```python
from build123d import *

# Parameters (mm, degrees)
SKETCH1_R          = 12.5
SKETCH1_R_2        = 1.5
SKETCH1_R_3        = 2.5
SKETCH1_R_4        = 2.25
BASE_FLANGE1_DEPTH = 1


# Sheet-metal steps are written as plain solids
with BuildPart() as part:
    # Sketch1 → Base-Flange1 (new body)
    with BuildSketch(Plane.XY):
        Polygon((-90.1, -21), (-48.1, -21), (-30.1, -50), (-20.1, -50), (4.727586207, -10), (90.1, -10), (90.1, 10), (4.727586207, 10), (-20.1, 50), (-30.1, 50), (-48.1, 21), (-90.1, 21), align=None)
        with Locations((-69.1, 0)):
            Circle(SKETCH1_R, mode=Mode.SUBTRACT)
        with Locations((-84.6, 15.5)):
            Circle(SKETCH1_R_2, mode=Mode.SUBTRACT)
        with Locations((-25.1, -40)):
            Circle(SKETCH1_R_3, mode=Mode.SUBTRACT)
        with Locations((80.1, 0)):
            Circle(SKETCH1_R_4, mode=Mode.SUBTRACT)
        with Locations((65.1, 0)):
            Circle(SKETCH1_R_4, mode=Mode.SUBTRACT)
        with Locations((25.1, 0)):
            Circle(SKETCH1_R_4, mode=Mode.SUBTRACT)
        with Locations((5.1, 0)):
            Circle(SKETCH1_R_4, mode=Mode.SUBTRACT)
        with Locations((36.1, 0)):
            Circle(SKETCH1_R_3, mode=Mode.SUBTRACT)
        with Locations(Location((-25.1, 40, 0), (0, 0, 180))):
            Circle(SKETCH1_R_3, mode=Mode.SUBTRACT)
        with Locations((-15.1, 0)):
            Circle(SKETCH1_R_4, mode=Mode.SUBTRACT)
        with Locations((-35.1, 0)):
            Circle(SKETCH1_R_4, mode=Mode.SUBTRACT)
        with Locations((-53.6, 15.5)):
            Circle(SKETCH1_R_2, mode=Mode.SUBTRACT)
        with Locations((-53.6, -15.5)):
            Circle(SKETCH1_R_2, mode=Mode.SUBTRACT)
        with Locations((-84.6, -15.5)):
            Circle(SKETCH1_R_2, mode=Mode.SUBTRACT)
    extrude(amount=-BASE_FLANGE1_DEPTH)


solid = part.part
```
Source: CAD feature listing. Evaluate the final solid. Frame: model axes, mm. Give positions to 0.01 mm unless a question says otherwise; leave off trailing zeros. Loops run counter-clockwise (first coordinate to the right, second up) from the corner with the lowest first, then second, coordinate; pieces in that order, holes last. Notation, with made-up numbers: (20.25, -10.75) - (78.25, -10.75) arc R25 ccw to (78.25, 2.25) - close; hole circle Ø1 at (9, 72.25). An arc over 180 degrees is marked (long way). Use CSV: the item, a comma, the result in double quotes. Start each with the question number.
1. Ray query, L1, parallel to Y at x = -25.1, z = -0.25; L2, parallel to Y at x = 57, z = -0.6; L3, parallel to Y at x = -35.1, z = -0.75. Return the intervals inside material, ascending.
2. Section C-C (x = 65.1). Output: boundary loops of the cut face in (y, z).
3. Pin query (flat end, axial travel): pin 1 (0.5 mm diameter, centred on x = -76.5, z = -0.5, fed in from -Y). Return the tip coordinate at first contact, or that it passes through.
4. Section B-B (z = -0.55). Count the separate pieces of the cut face and the enclosed holes in it, then the cut area to 3 significant figures.
5. Section A-A (x = -25.1). Output: boundary loops of the cut face in (y, z), then the cut area to 3 significant figures.
6. Section D-D (y = 40). Output: boundary loops of the cut face in (x, z).
7. Draft query along X for faces 1 (the cylindrical face through (27.246, 0.676, -0.493)), 2 (the flat face through (-38.974, 35.703, -0.493)), 3 (the flat face through (-7.5, 29.7, -0.5)), 4 (the flat face through (-20, 0, -1)). Return one class per face: +X half, -X half, draft (parallel to the pull), parting line (faces both ways), or undercut.
Response:
1,L1,"-50 to -42.5, -37.5 to 37.5, 42.5 to 50"
1,L2,"-10 to 10"
1,L3,"-41.94 to -2.25, 2.25 to 41.94"
2,outline,"(-10, -1) - (-2.25, -1) - (-2.25, 0) - (-10, 0) - close; (2.25, -1) - (10, -1) - (10, 0) - (2.25, 0) - close"
3,pin 1,"y = -21"
4,separate pieces,"1"
4,enclosed holes,"14"
4,area,"6,570 mm²"
5,outline,"(-50, -1) - (-42.5, -1) - (-42.5, 0) - (-50, 0) - close; (-37.5, -1) - (37.5, -1) - (37.5, 0) - (-37.5, 0) - close; (42.5, -1) - (50, -1) - (50, 0) - (42.5, 0) - close"
5,area,"90.0 mm²"
6,outline,"(-36.31, -1) - (-27.6, -1) - (-27.6, 0) - (-36.31, 0) - close; (-22.6, -1) - (-13.89, -1) - (-13.89, 0) - (-22.6, 0) - close"
7,face 1,"undercut"
7,face 2,"-X half"
7,face 3,"+X half"
7,face 4,"draft"
